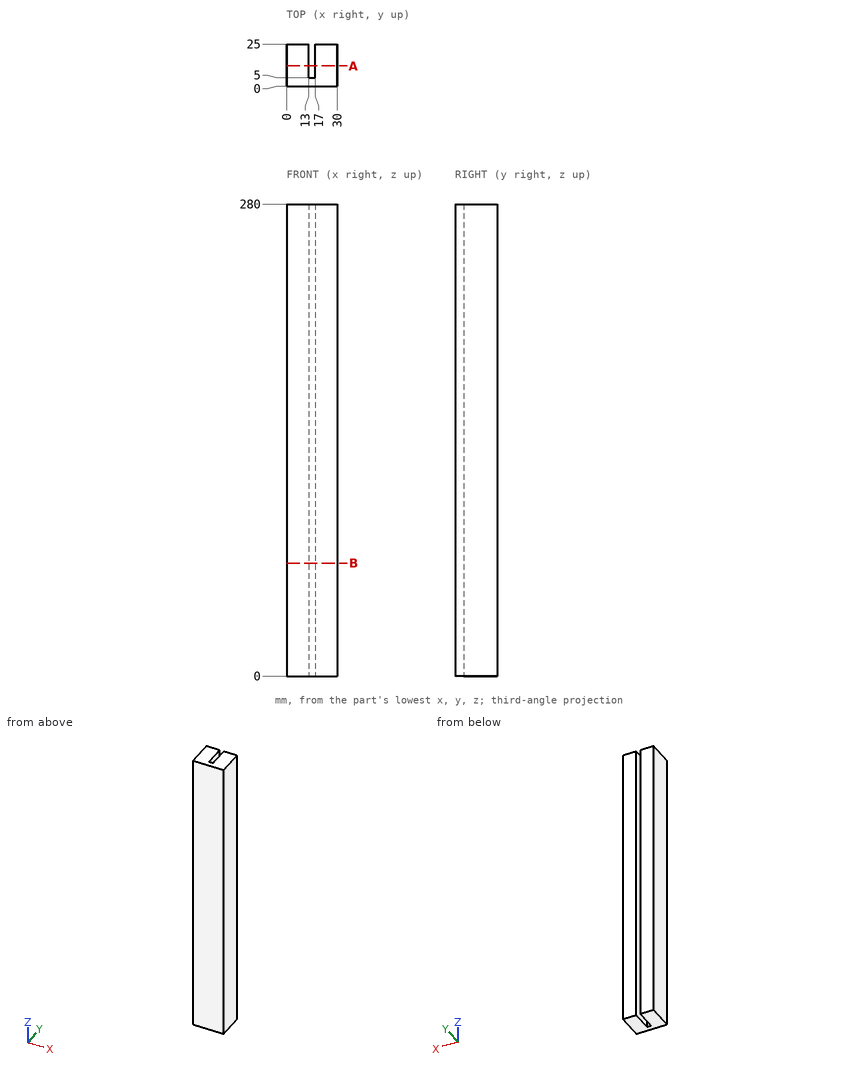
Job drawing, mm, ordinate dimensions from the low corner. One solid piece. Round coordinates to 2 decimals unless told otherwise and drop trailing zeros. Loops run counter-clockwise (first coordinate to the right, second up) from the corner with the lowest first, then second, coordinate; pieces in that order, holes last.
(1) Cut at A-A (y = 12). Give the cut face in (x, z), plus the area to 3 significant figures.
(2) Cut at B-B (z = 67). Give the cut face in (x, y).
(3) Drop flat-ended pins along their axis: pin 1 (5 mm diameter, centred on y = 3, z = 242.5, fed in from -X); pin 2 (2 mm diameter, centred on x = 15.5, z = 76.5, fed in from +Y). Give the stop position or say it passes through.
(4) Wall check: line 1 along X through (y, z) = (19, 127.5); line 2 along Y through (x, z) = (13.5, 142). Give the ranges that are in metal, low to high.
Findings below:
1. outline: (0, 0) - (13, 0) - (13, 280) - (0, 280) - close; (17, 0) - (30, 0) - (30, 280) - (17, 280) - close
1. area: 7,280 mm2
2. outline: (0, 0) - (30, 0) - (30, 25) - (17, 25) - (17, 5) - (13, 5) - (13, 25) - (0, 25) - close
3. pin 1: stops at x = 0
3. pin 2: stops at y = 5
4. line 1: x = 0 to 13, 17 to 30
4. line 2: y = 0 to 5
